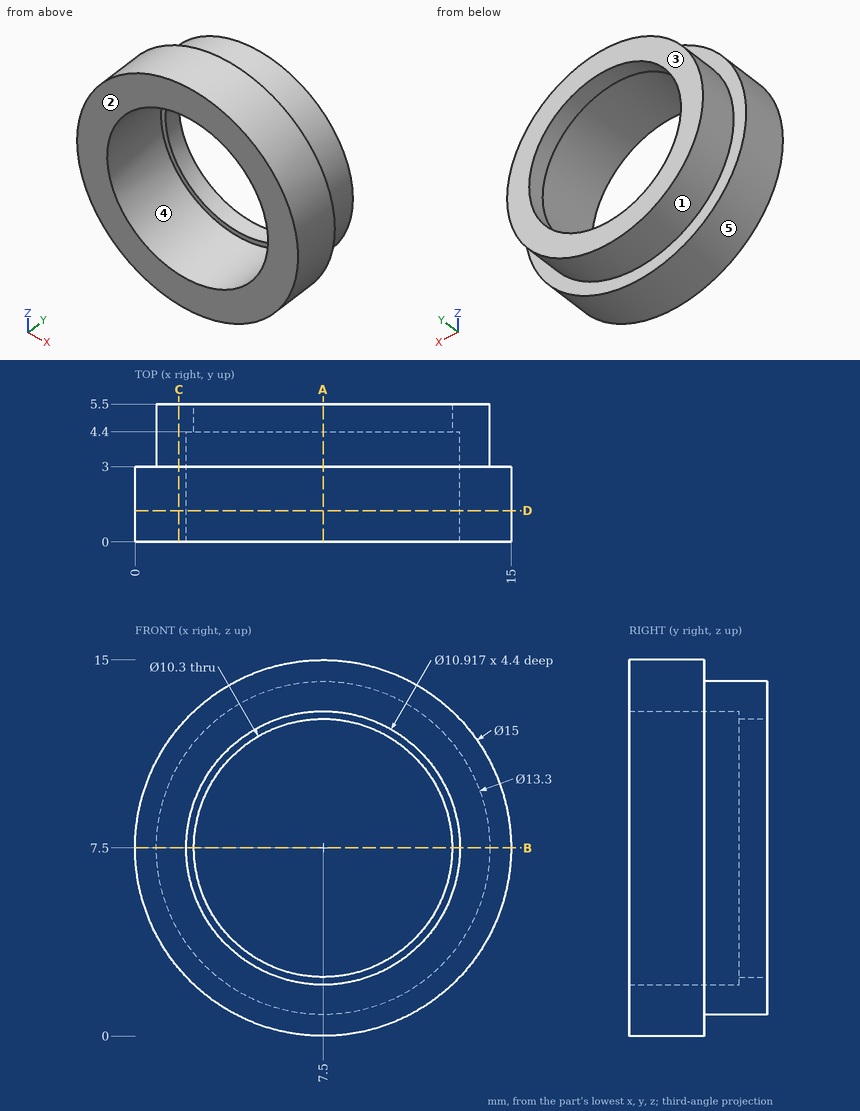
Study the drawing (mm; zero at the part's minimum x, y, z) and answer. A direction names the side the tool comes from. Give positions to 0.01 mm unless a question says otherwise; leave off trailing zeros. Write each loop counter-clockwise with the first axis right and the second up, starting at its lowest first coordinate (ties: lowest second). Pieces come first, ordered by that corner, then holes.
Item 1: Which of the six approach directions +Z, -Z, +X, -X, +Y, -Y give full straight-line access (tool end or side, diameter ignored) to the marked faces 1 and 2?
Item 2: Section A-A, the plane x = 7.5 is taken. Write down the section's boundary in (y, z).
Item 3: Determine the mould class of the marked faces 3, 4 and 5 for opening direction Z: released by +Z, released by -Z, zero draft, split by the parting line, or undercut.
Item 4: Section B-B, the plane z = 7.5 is taken. Write down the section's boundary in (x, y), plus the area to 3 significant figures.
Item 5: Find the intervals of material crossed by line 1 along X through (y, z) = (3.5, 7.5); line 2 along X through (y, z) = (5.1, 7.5), in increasing order.
Item 6: Section D-D, the plane y = 1.25 is taken. Write down the section's boundary in (x, z), plus the area to 3 significant figures.
Item 7: Flat-ended cylindrical pins translate along their axes: P1, Ø1, axis at y = 2, z = 5, coming from the -X side; P2, Ø2, axis at x = 11, y = 3, coming from the +Z side; P3, Ø2, axis at x = 8.5, z = 5.5, coming from the +Y side. Find the tip coordinate at first contact, or state that the pin passes through.
Item 8: Section C-C, the plane x = 1.75 is taken. Write down the section's boundary in (y, z), plus the area to 3 significant figures.
Completed:
1. face 1: +Y
1. face 2: +Z, -Z, +X, -X, -Y
2. outline: (0, 0) - (3, 0) - (3, 0.85) - (5.5, 0.85) - (5.5, 2.35) - (4.4, 2.35) - (4.4, 2.04) - (0, 2.04) - close; (0, 12.96) - (4.4, 12.96) - (4.4, 12.65) - (5.5, 12.65) - (5.5, 14.15) - (3, 14.15) - (3, 15) - (0, 15) - close
3. face 3: zero draft
3. face 4: undercut
3. face 5: split by the parting line
4. outline: (0, 0) - (2.04, 0) - (2.04, 4.4) - (2.35, 4.4) - (2.35, 5.5) - (0.85, 5.5) - (0.85, 3) - (0, 3) - close; (12.65, 4.4) - (12.96, 4.4) - (12.96, 0) - (15, 0) - (15, 3) - (14.15, 3) - (14.15, 5.5) - (12.65, 5.5) - close
4. area: 18.9 mm2
5. line 1: x = 0.85 to 2.04, 12.96 to 14.15
5. line 2: x = 0.85 to 2.35, 12.65 to 14.15
6. outline: circle Ø15 at (7.5, 7.5); hole circle Ø10.92 at (7.5, 7.5)
6. area: 83.1 mm2
7. P1: stops at x = 0.27
7. P2: stops at z = 14.57
7. P3: passes through
8. outline: (0, 2.68) - (3, 2.68) - (3, 4.16) - (5.5, 4.16) - (5.5, 10.84) - (3, 10.84) - (3, 12.32) - (0, 12.32) - close
8. area: 45.6 mm2
